Study the drawing (mm; zero at the part's minimum x, y, z) and answer. A direction names the side the tool comes from. Give positions to 0.01 mm unless a question says otherwise; leave off trailing zeros. Loops run counter-clockwise (first coordinate to the right, second up) from the corner with the lowest first, then second, coordinate; pieces in that order, holes last. Notation, with made-up numbers: (7, 62) - (41, 62) arc R36 cw to (41, 96) - close; hole circle Ø10 at (18.25, 11). An arc over 180 degrees is marked (long way). Answer in a Markdown table with one row per item. Add a question column.
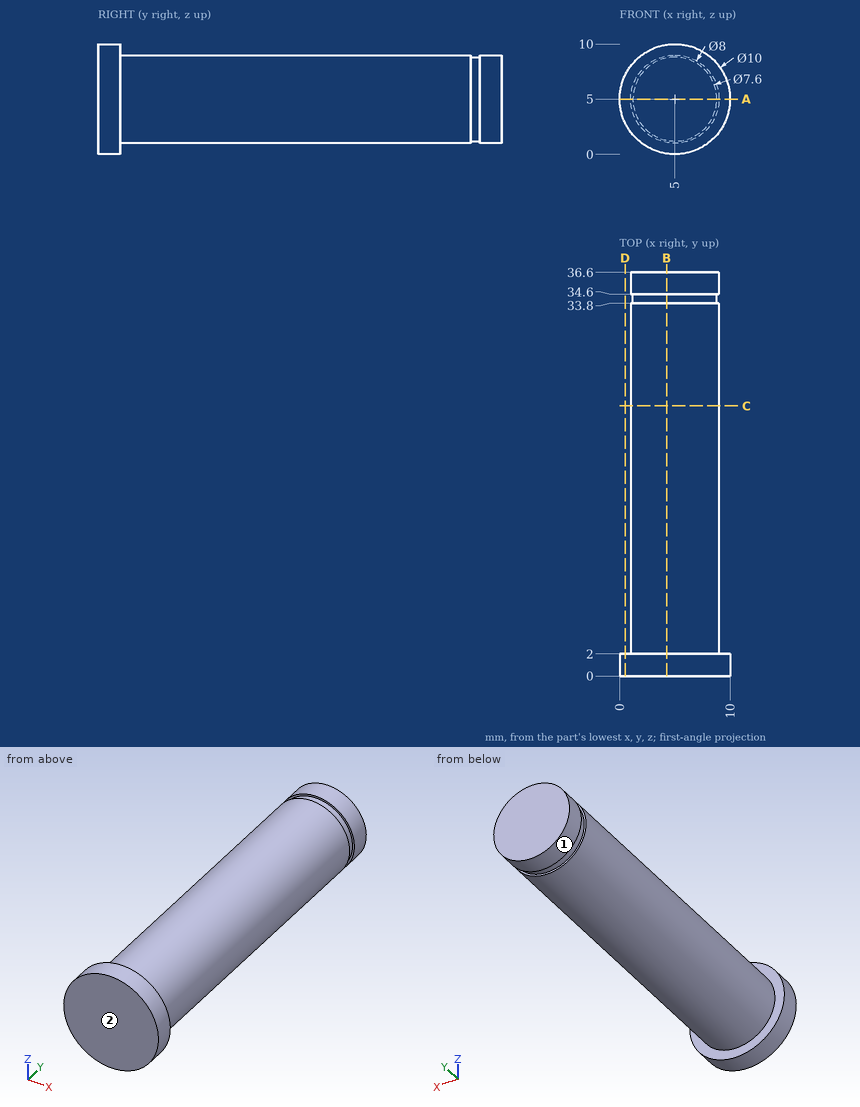
(1) A cutting plane is placed at D-D on x = 0.5. Determine the outline of the cut face in (y, z).
(2) A cutting plane is placed at A-A on z = 5. Determine the outline of the cut face in (x, y), plus the area to 3 significant figures.
(3) A tool of negligible diameter and unlimited length cuts with its end or side. For the marked faces 1 and 2, from which of +Z, -Z, +X, -X, +Y, -Y can it reach the whole face along a straight path? Write none if from no direction.
(4) A cutting plane is placed at B-B on x = 4.25. Determine the outline of the cut face in (y, z).
(5) Find the intervals of material crossed by line 1 along Y through (x, z) = (2, 2.5); line 2 along X through (y, z) = (5.5, 5); line 3 along Y through (x, z) = (9, 2.25), in increasing order. Write a range as [from, to].
(6) Given pin 1 Ø4 at (x, y) = (1.5, 10) entering from +Z; pin 2 Ø2 at (x, z) = (1.5, 6) entering from -Y; pin 3 Ø6 at (y, z) = (8, 5) entering from -X; pin 4 Ø1 at (y, z) = (16.5, 7) entering from +X, each flat-ended and moving along its own axis, determine where each tip first touches the part or whether it passes through.
(7) A cutting plane is placed at C-C on y = 24.5. Determine the outline of the cut face in (x, z), plus the area to 3 significant figures.
Evaluation:
| question | item | result |
|---|---|---|
| 1 | outline | (0, 2.82) - (2, 2.82) - (2, 7.18) - (0, 7.18) - close |
| 2 | outline | (0, 0) - (10, 0) - (10, 2) - (9, 2) - (9, 33.8) - (8.8, 33.8) - (8.8, 34.6) - (9, 34.6) - (9, 36.6) - (1, 36.6) - (1, 34.6) - (1.2, 34.6) - (1.2, 33.8) - (1, 33.8) - (1, 2) - (0, 2) - close |
| 2 | area | 296 mm² |
| 3 | face 1 | +Y |
| 3 | face 2 | +Z, -Z, +X, -X, -Y |
| 4 | outline | (0, 0.06) - (2, 0.06) - (2, 1.07) - (33.8, 1.07) - (33.8, 1.27) - (34.6, 1.27) - (34.6, 1.07) - (36.6, 1.07) - (36.6, 8.93) - (34.6, 8.93) - (34.6, 8.73) - (33.8, 8.73) - (33.8, 8.93) - (2, 8.93) - (2, 9.94) - (0, 9.94) - close |
| 5 | line 1 | y = [0, 33.8], [34.6, 36.6] |
| 5 | line 2 | x = [1, 9] |
| 5 | line 3 | y = [0, 2] |
| 6 | pin 1 | stops at z = 8.71 |
| 6 | pin 2 | stops at y = 0 |
| 6 | pin 3 | stops at x = 1 |
| 6 | pin 4 | stops at x = 8.71 |
| 7 | outline | circle Ø8 at (5, 5) |
| 7 | area | 50.3 mm² |
